Design review of the part shown in the three views and the two pictorial views. Dimensions are in mm from the part's minimum x, y and z. Coordinates: 2 decimals unless noted, no trailing zeros. Write each loop counter-clockwise with the first axis right and the second up, starting at its lowest first coordinate (ties: lowest second). Pieces come first, ordered by that corner, then holes.
Q1. Take a section at D-D, the plane x = 18.5. Write out the cut boundary in (y, z), plus the area to 3 significant figures.
Q2. Take a section at C-C, the plane y = 4. Write out the cut boundary in (x, z), plus the area to 3 significant figures.
Q3. For L1, parallel to Y at x = 27, z = 0.45 (1 decimal); L2, parallel to Y at x = 21, z = 1.2; L3, parallel to X at y = 8, z = 0.7 (1 decimal), list the stretches that pass through material, from the lowest coordinate up.
Q4. Take a section at A-A, the plane z = 1.3. Write out the cut boundary in (x, y) (1 decimal).
Q5. For pin 1 Ø0.5 at (y, z) = (1.5, 1) entering from -X; pin 2 Ø0.5 at (y, z) = (2, 0.5) entering from +X; pin 3 Ø1.6 at (x, y) = (7, 27.23) entering from -Z; pin 4 Ø0.5 at (x, z) = (14.5, 1) entering from -Y, all flat-tipped, find the tip position at first contact; note any pin that passes through.
Q6. Take a section at B-B, the plane x = 27. Write out the cut boundary in (y, z), plus the area to 3 significant figures.
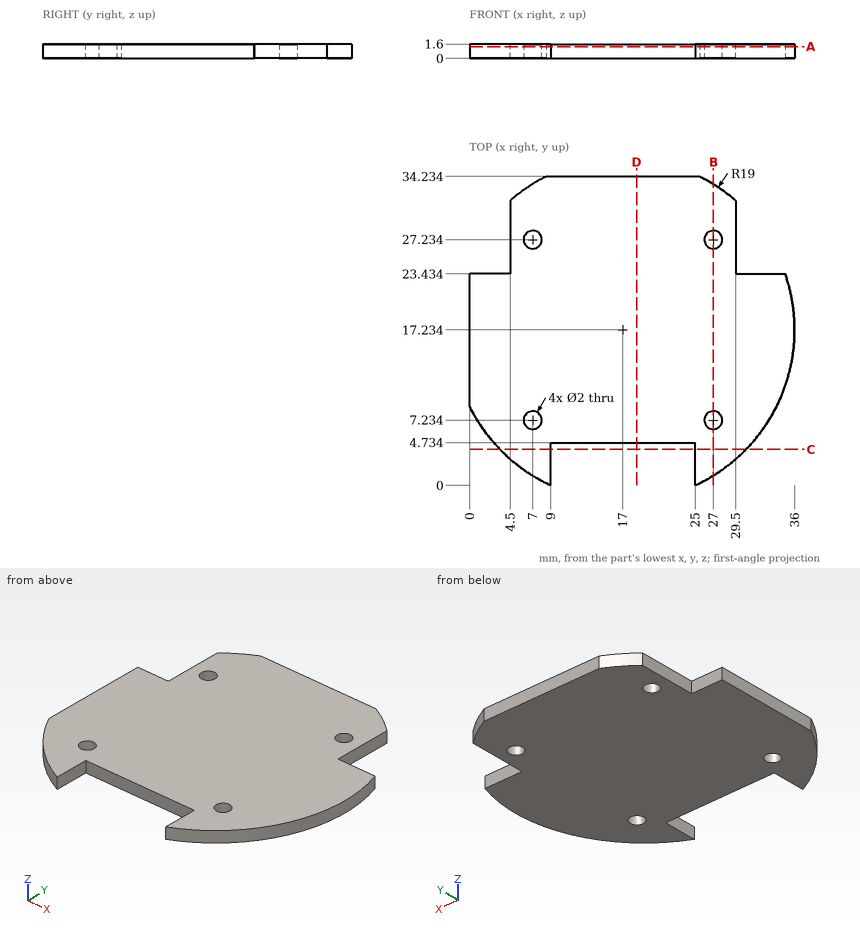
Responses:
1. outline: (4.73, 0) - (34.23, 0) - (34.23, 1.6) - (4.73, 1.6) - close
1. area: 47.2 mm2
2. outline: (3.37, 0) - (9, 0) - (9, 1.6) - (3.37, 1.6) - close; (25, 0) - (30.63, 0) - (30.63, 1.6) - (25, 1.6) - close
2. area: 18.0 mm2
3. L1: y = 1.1 to 6.2, 8.2 to 26.2, 28.2 to 33.4
3. L2: y = 4.73 to 34.23
3. L3: x = 0.4 to 6.4, 7.6 to 26.4, 27.6 to 33.6
4. outline: (0, 8.7) arc R19 ccw to (9, 0) - (9, 4.7) - (25, 4.7) - (25, 0) arc R19 ccw to (35, 23.4) - (29.5, 23.4) - (29.5, 31.5) arc R19 ccw to (25.5, 34.2) - (8.5, 34.2) arc R19 ccw to (4.5, 31.5) - (4.5, 23.4) - (0, 23.4) - close; hole circle Ø2 at (7, 7.2); hole circle Ø2 at (7, 27.2); hole circle Ø2 at (27, 7.2); hole circle Ø2 at (27, 27.2)
5. pin 1: stops at x = 5.99
5. pin 2: stops at x = 28.68
5. pin 3: passes through
5. pin 4: stops at y = 4.73
6. outline: (1.08, 0) - (6.23, 0) - (6.23, 1.6) - (1.08, 1.6) - close; (8.23, 0) - (26.23, 0) - (26.23, 1.6) - (8.23, 1.6) - close; (28.23, 0) - (33.39, 0) - (33.39, 1.6) - (28.23, 1.6) - close
6. area: 45.3 mm2
